Design review of the part shown in the three views and the two pictorial views. Dimensions are in mm from the part's minimum x, y and z. Give positions to 0.01 mm unless a question says otherwise; leave off trailing zeros. Order: outer loops, then holes, each group sorted by start corner. A loop starts at its lowest first (then second) coordinate and runs counter-clockwise, first axis right, second up. Notation, with made-up numbers: (-18.5, 78.5) - (40.5, 78.5) arc R9 cw to (40.5, 90.5) - close; hole circle Ø9 at (4.25, 49.25). An arc over 180 degrees is marked (long way). Put each result on its own line as item: value. Start each with the question number.
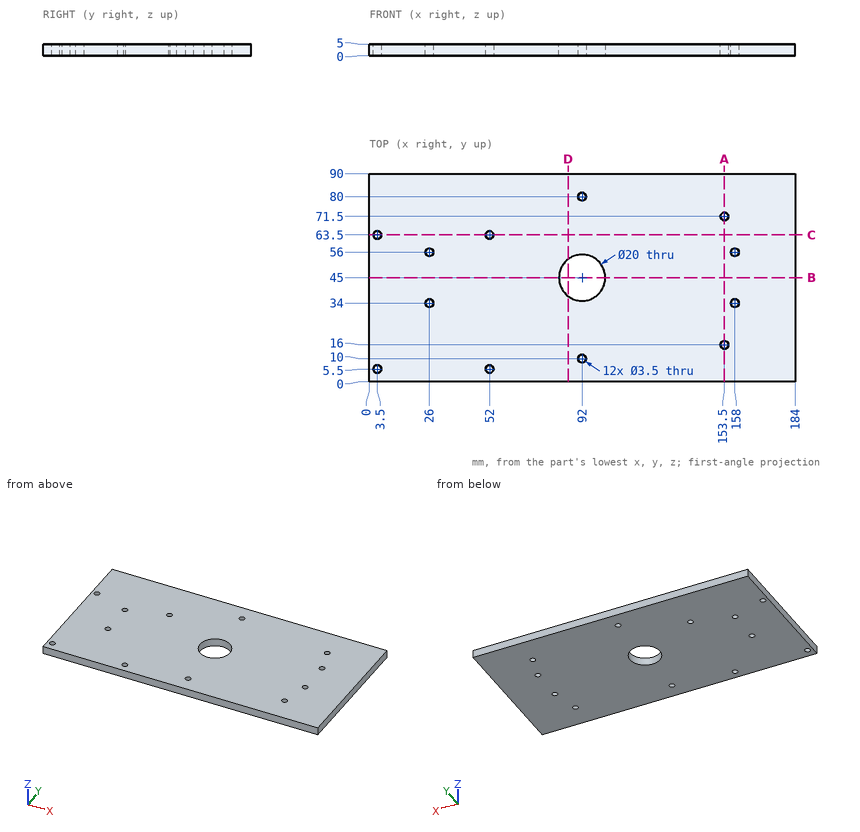
1. Add section A-A, the plane x = 153.5. Give the boundary of the cut face in (y, z).
2. Add section B-B, the plane y = 45. Give the boundary of the cut face in (x, z).
3. Add section C-C, the plane y = 63.5. Give the boundary of the cut face in (x, z).
4. Wall thickness on line 1 (X direction, y = 63.5, z = 3.85); line 2 (Y direction, x = 3.5, z = 3.05); line 3 (Y direction, x = 153.5, z = 1.8): over which ranges is each line inside the solid? List them lowest first. Write a range as from..to.
5. Clearance check with a flat-ended pin moving along its axis: pin 1 (2 mm diameter, centred on x = 3.5, y = 5.5, fed in from +Z) (3 decimals). State where the tip first meets the part, or that it passes through.
6. Add section D-D, the plane x = 86. Give the boundary of the cut face in (y, z), then the cut area to 3 significant figures.
Found:
1. outline: (0, 0) - (14.25, 0) - (14.25, 5) - (0, 5) - close; (17.75, 0) - (69.75, 0) - (69.75, 5) - (17.75, 5) - close; (73.25, 0) - (90, 0) - (90, 5) - (73.25, 5) - close
2. outline: (0, 0) - (82, 0) - (82, 5) - (0, 5) - close; (102, 0) - (184, 0) - (184, 5) - (102, 5) - close
3. outline: (0, 0) - (1.75, 0) - (1.75, 5) - (0, 5) - close; (5.25, 0) - (50.25, 0) - (50.25, 5) - (5.25, 5) - close; (53.75, 0) - (184, 0) - (184, 5) - (53.75, 5) - close
4. line 1: x = 0..1.75, 5.25..50.25, 53.75..184
4. line 2: y = 0..3.75, 7.25..61.75, 65.25..90
4. line 3: y = 0..14.25, 17.75..69.75, 73.25..90
5. pin 1: passes through
6. outline: (0, 0) - (37, 0) - (37, 5) - (0, 5) - close; (53, 0) - (90, 0) - (90, 5) - (53, 5) - close
6. area: 370 mm^2
